Read the model definition and answer for the solid it produces. Units are mm, in the model's axes. Face numbers are marked on the shaded views. Round coordinates to 2 decimals unless told otherwise and drop trailing zeros. Order: outer loops, then holes, each group sorted by start corner. A loop starts at its lowest first (then second) coordinate and runs counter-clockwise, first axis right, second up.
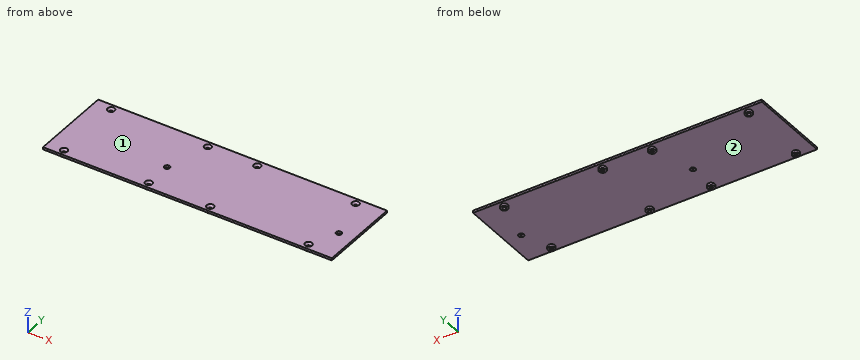
Autodesk Inventor part; units mm, degrees
ref_plane "YZ Plane" through (0, 0, 0) normal (1, 0, 0) x (0, 1, 0)
ref_plane "XZ Plane" through (0, 0, 0) normal (0, 1, 0) x (-1, 0, 0)
ref_plane "XY Plane" through (0, 0, 0) normal (0, 0, 1) x (1, 0, 0)
sketch "Sketch1" plane through (0, 0, 0) normal (0, 0, 1) x (1, 0, 0)
  line L0 (-138.811, 39.7129) -> (138.811, 39.7129)
  line L1 (138.811, 39.7129) -> (138.811, -39.7129)
  line L2 (138.811, -39.7129) -> (-138.811, -39.7129)
  line L3 (-138.811, -39.7129) -> (-138.811, 39.7129)
  line L4 (0, 0) -> (0, 39.7129) construction
  line L5 (0, 0) -> (0, -39.7129) construction
  line L6 (0, 0) -> (-138.811, 0) construction
  line L7 (0, 0) -> (138.811, 0) construction
  dimension "d0" = 277.622
  dimension "d1" = 79.4258
extrude "Extrusion1" add sketch "Sketch1" along normal mid plane 2.2098
sketch "Sketch2" plane through (0, 0, 1.1049) normal (0, 0, 1) x (1, 0, 0)
  line L0 (138.811, 39.7129) -> (138.811, -39.7129)
  line L1 (-138.811, 39.7129) -> (138.811, 39.7129)
  line L2 (-138.811, -39.7129) -> (-138.811, 39.7129)
  line L3 (138.811, -39.7129) -> (-138.811, -39.7129)
  circle A0 centre (-122.5042, 33.9217) radius 3.3401
  circle A1 centre (-29.4894, 33.9217) radius 3.3401
  circle A2 centre (18.0848, 33.9217) radius 3.3401
  circle A3 centre (112.5728, 33.9217) radius 3.3401
  circle A4 centre (-122.5042, -33.9217) radius 3.3401
  circle A5 centre (-40.9702, -33.9217) radius 3.3401
  circle A6 centre (18.0848, -33.9217) radius 3.3401
  circle A7 centre (112.5728, -33.9217) radius 3.3401
  dimension "d4" = 16.3068
  dimension "d5" = 5.7912
  dimension "d6" = 5.7912
  dimension "d7" = 26.2382
  dimension "d8" = 120.7262
  dimension "d9" = 168.3004
  dimension "d10" = 179.7812
  dimension "d11" = 6.6802
extrude "Extrusion2" add sketch "Sketch2" against normal blind 4.5974 contours A0 | A1 | A2 | A3 | A4 | A5 | A6 | A7
sketch "Sketch3" plane through (0, 0, 1.1049) normal (0, 0, 1) x (1, 0, 0)
  circle A0 centre (-122.5042, 33.9217) radius 3.3401
  circle A1 centre (-122.5042, -33.9217) radius 3.3401
  circle A2 centre (-29.4894, 33.9217) radius 3.3401
  circle A3 centre (-40.9702, -33.9217) radius 3.3401
  circle A4 centre (18.0848, -33.9217) radius 3.3401
  circle A5 centre (18.0848, 33.9217) radius 3.3401
  circle A6 centre (112.5728, 33.9217) radius 3.3401
  circle A7 centre (112.5728, -33.9217) radius 3.3401
hole "Hole1" at (-122.5042, 33.9217, 1.1049) at (-29.4894, 33.9217, 1.1049) at (18.0848, 33.9217, 1.1049) at (112.5728, 33.9217, 1.1049) at (112.5728, -33.9217, 1.1049) at (18.0848, -33.9217, 1.1049) at (-40.9702, -33.9217, 1.1049) at (-122.5042, -33.9217, 1.1049) direction (0, 0, -1) diameter 3.1496 end through all countersink diameter 6.731 countersink angle 82
sketch "Sketch4" plane through (0, 0, 1.1049) normal (0, 0, 1) x (1, 0, 0)
  line L0 (138.811, 39.7129) -> (138.811, -39.7129)
  line L1 (-138.811, 39.7129) -> (138.811, 39.7129)
  point P0 (-40.9702, -7.6581)
  point P1 (124.1298, -7.6581)
  dimension "d21" = 47.371
  dimension "d22" = 14.6812
  dimension "d23" = 165.1
hole "Hole2" at (-40.9702, -7.6581, 1.1049) at (124.1298, -7.6581, 1.1049) direction (0, 0, -1) diameter 5.2324 end through all
properties part number "cRIO-FRC BackPlate" material "Aluminum-Casting"
Q1. For a pull along X with two mould halves and no side action, classify the marked faces 1 and 2 as released by +X, released by -X, zero draft, split by the parting line, or undercut.
Outcome:
face 1: zero draft
face 2: undercut
Q2. A cutting plane is placed at A-A, the plane z = -2.5. Give the number of separate pieces and of enclosed holes in the cut face, plus the area to 3 significant figures.
Outcome:
separate pieces: 8
enclosed holes: 8
area: 218 mm2
Q3. A cutting plane is placed at B-B, the plane y = -20. Give the vertices of the cut face in (x, z).
Outcome:
outline: (-138.81, -1.1) - (138.81, -1.1) - (138.81, 1.1) - (-138.81, 1.1) - close
Q4. A cutting plane is placed at C-C, the plane x = 64.5. Give the vertices of the cut face in (y, z), plus the area to 3 significant figures.
Outcome:
outline: (-39.71, -1.1) - (39.71, -1.1) - (39.71, 1.1) - (-39.71, 1.1) - close
area: 176 mm2
Q5. Straight lines are drawn through the part: probe 1 along Y at (x, z) = (-41, -1.3); probe 2 along X at (y, z) = (-34.5, 0.9); probe 3 along Z at (x, y) = (11.5, 27.5). For each, find the intervals that lie inside material, in ascending order.
Outcome:
probe 1: y = -37.26 to -35.5, -32.35 to -30.58
probe 2: x = -138.81 to -125.64, -119.37 to -44.1, -37.84 to 14.95, 21.22 to 109.44, 115.71 to 138.81
probe 3: z = -1.1 to 1.1
Q6. Flat-ended cylindrical pins translate along their axes: pin 1 (8.5 mm diameter, centred on x = 124.13, y = -7.66, fed in from -Z); pin 2 (5 mm diameter, centred on x = 18.08, y = 33.92, fed in from +Z); pin 3 (4 mm diameter, centred on x = 112.57, y = -33.92, fed in from +Z). Find the tip coordinate at first contact, or state that the pin passes through.
Outcome:
pin 1: stops at z = -1.1
pin 2: stops at z = 0.12
pin 3: stops at z = -0.46
